Design review of the part built by this model. Coordinates are the model's own, in mm. A direction names the side the tool comes from. Coordinates: 2 decimals unless noted, no trailing zeros. Order: outer loops, then holes, each group sorted by start corner. A loop starts at its lowest first (then second) coordinate and runs counter-clockwise, first axis right, second up. Notation, with made-up numbers: M 1,7 L 30,7 A15 ccw 30,24 Z; hole C -17.75,68.25 d5. An arc over 180 degrees is marked long. Answer in a Markdown table with one row per item.
from build123d import *

# Parameters (mm, degrees)
F0_W     = 50.147576
F0_H     = 34.925
F0_R     = 1.7272
F0_R_2   = 11.1125
F1_DEPTH = 6.35
F2_W     = 28.575
F2_H     = 28.575
F2_R     = 11.1125
F3_DEPTH = 9.525
F4_R     = 1.7272
F5_DEPTH = 28.575
F6_R     = 9.525


with BuildPart() as f1:
    # F0 (on Top) → F1 (new body)
    with BuildSketch(Plane.XY):
        Rectangle(F0_W, F0_H)
        with Locations((-20.311288, -12.7)):
            Circle(F0_R, mode=Mode.SUBTRACT)
        with Locations((20.311288, -12.7)):
            Circle(F0_R, mode=Mode.SUBTRACT)
        with Locations((-20.311288, 12.7)):
            Circle(F0_R, mode=Mode.SUBTRACT)
        Circle(F0_R_2, mode=Mode.SUBTRACT)
        with Locations((20.311288, 12.7)):
            Circle(F0_R, mode=Mode.SUBTRACT)
    extrude(amount=F1_DEPTH)

    # F2 (on face) → F3 (join)
    with BuildSketch(Plane.XY.offset(6.35)):
        Rectangle(F2_W, F2_H)
        Circle(F2_R, mode=Mode.SUBTRACT)
    extrude(amount=F3_DEPTH)

    # F4 (on face) → F5 (cut, through all)
    with BuildSketch(Plane(origin=(0, 14.2875, 0), x_dir=(-1, 0, 0), z_dir=(0, 1, 0))):
        with Locations((0, 11.1125)):
            Circle(F4_R)
    extrude(amount=-F5_DEPTH, mode=Mode.SUBTRACT)

    # F6
    f6_edges = [f1.edges().sort_by_distance(p)[0] for p in [
        (-14.2875, -14.2875, 11.1125),
        (14.2875, -14.2875, 11.1125),
        (14.2875, 14.2875, 11.1125),
        (-14.2875, 14.2875, 11.1125),
    ]]
    fillet(f6_edges, radius=F6_R)


solid = f1.part
(1) Add section C-C, the plane z = 5.5. Give the boundary of the cut face in (x, y) (1 decimal), and give its area (3 significant figures).
Return value:
| item | result |
|---|---|
| outline | M -25.1,-17.5 L 25.1,-17.5 L 25.1,17.5 L -25.1,17.5 Z; hole C -20.3,-12.7 d3.5; hole C -20.3,12.7 d3.5; hole C 0,0 d22.2; hole C 20.3,-12.7 d3.5; hole C 20.3,12.7 d3.5 |
| area | 1,330 mm2 |
(2) Draft analysis for pull direction Y (two halves, no side actions). For faces 5 (the flat face through (2, 14.288, 11)), 6 (the cylindrical face through (21.96, -12.18, 3.13)), 7 (the cylindrical face through (0.225, 12.654, 12.825)), state which applies: pulls with the +Y half, pulls with the -Y half, needs draft (parallel to the pull), parting line crosses it, or undercut.
Return value:
| item | result |
|---|---|
| face 5 | pulls with the +Y half |
| face 6 | undercut |
| face 7 | needs draft |
(3) Insertion check: pin 1 Ø4 at (x, y) = (-20.31, -12.7) entering from +Z; pin 2 Ø3 at (y, z) = (1.5, 11) entering from +X; pin 3 Ø2 at (y, z) = (-13.5, 11.5) entering from -X. Each pin has a flat end and moves straight along its axis. Give the tip position at first contact, or say it passes through.
Return value:
| item | result |
|---|---|
| pin 1 | stops at z = 6.35 |
| pin 2 | stops at x = 14.29 |
| pin 3 | stops at x = -10.32 |
(4) For line 1 along X through (y, z) = (-0.5, 14.75); line 2 along Z through (x, y) = (7.5, 14.5), list the stretches that pass through material, from the lowest coordinate up. Write a range as from..to.
Return value:
| item | result |
|---|---|
| line 1 | x = -14.29..-11.1, 11.1..14.29 |
| line 2 | z = 0..6.35 |
(5) For faces 1 (the cylindrical face through (11.423, 11.571, 11.179)), 2 (the cylindrical face through (11.423, -11.571, 11.179)), 3 (the cylindrical face through (-11.571, -11.423, 11.179)), 4 (the flat face through (14.288, 0, 11)), list the 3-axis set-ups (+Z, -Z, +X, -X, +Y, -Y) from which the entire face can be reached by the end or side of a thin tool; tool diameter is ignored.
Return value:
| item | result |
|---|---|
| face 1 | +Z, +X, +Y |
| face 2 | +Z, +X, -Y |
| face 3 | +Z, -X, -Y |
| face 4 | +Z, +X, +Y, -Y |
(6) Add section A-A, the plane x = 0. Give the number of separate pieces and of enclosed holes in the cut face, and give its area (3 significant figures).
Return value:
| item | result |
|---|---|
| separate pieces | 4 |
| enclosed holes | 0 |
| area | 119 mm2 |
